Geometry: see drawing. Coordinates: mm, zero at the bounding-box minimum. A direction names the side the tool comes from. Coordinates: 2 decimals unless noted, no trailing zeros. Loops run counter-clockwise (first coordinate to the right, second up) from the corner with the lowest first, then second, coordinate; pieces in that order, holes last. Notation, with made-up numbers: (-23.5, -1.75) - (-10.5, -1.75) arc R14 ccw to (-10.5, 24.25) - close; hole circle Ø11 at (-10.75, 42). An arc over 180 degrees is marked (long way). Use a Markdown table: item, result. Add a question column.
1. Section query A-A on x = 36.65. Return the cut outline in (y, z).
2. Section query B-B on y = 26. Return the cut outline in (x, z).
3. Section query D-D on x = 21.15. Return the cut outline in (y, z), then the cut area to 3 significant figures.
4. Section query C-C on z = 36.65. Return the cut outline in (x, y).
5. Access query for the marked faces 1 and 2. Directions: +Z, -Z, +X, -X, +Y, -Y. A direction counts if a zero-diameter tool reaches every point of the face in a straight line with its end or side. Return the directions, or none.
6. Ray query, L1, parallel to Z at x = 36.65, y = 23.5; L2, parallel to X at y = 34, z = 7; L3, parallel to X at y = 23, z = 36. Return the intervals inside material, ascending. Write a range as [from, to].
7. Contact query for flat-ended pins moving along their axis: P1, Ø4, axis at x = 5.65, z = 36.65, coming from the -Y side; P2, Ø1.8, axis at x = 36.65, z = 36.65, coming from the -Y side; P3, Ø8, axis at x = 18.5, y = 11, coming from the -Z side. Output: stop coordinate, or through.
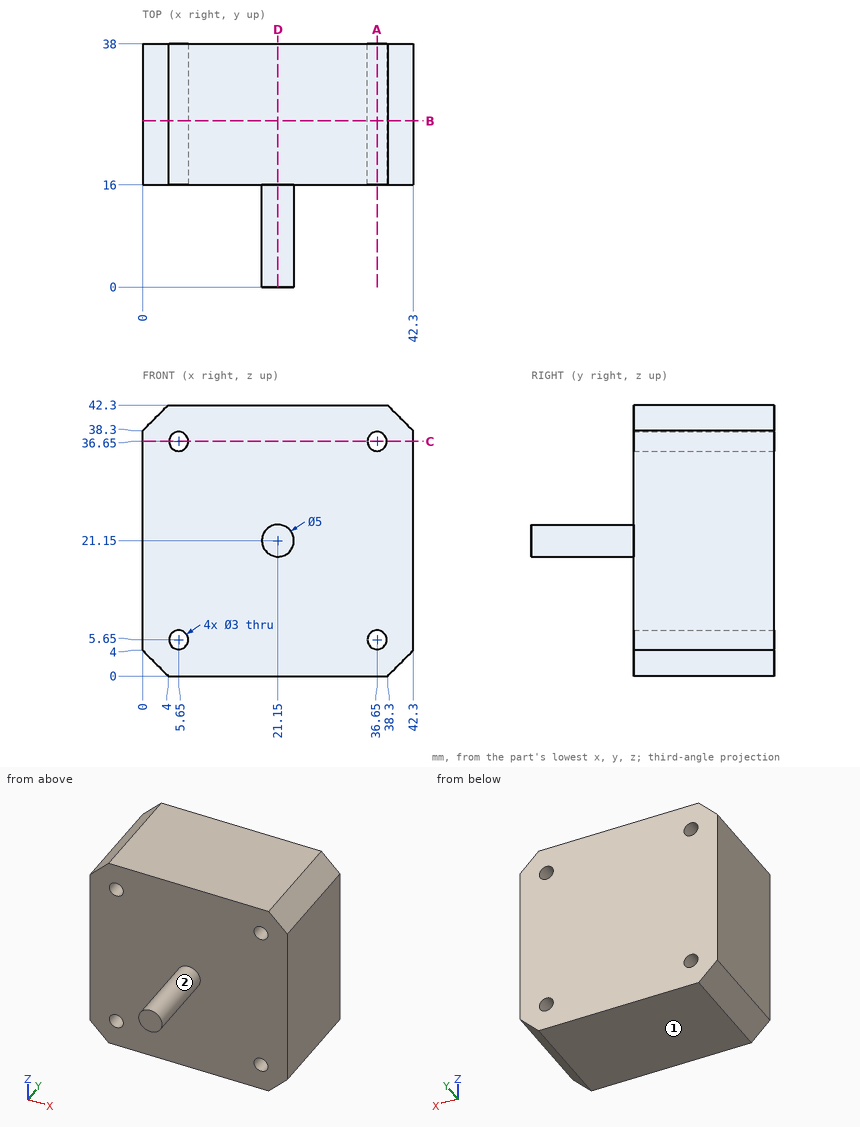
Resolved:
| question | item | result |
|---|---|---|
| 1 | outline | (16, 0) - (38, 0) - (38, 4.15) - (16, 4.15) - close; (16, 7.15) - (38, 7.15) - (38, 35.15) - (16, 35.15) - close; (16, 38.15) - (38, 38.15) - (38, 42.3) - (16, 42.3) - close |
| 2 | outline | (0, 4) - (4, 0) - (38.3, 0) - (42.3, 4) - (42.3, 38.3) - (38.3, 42.3) - (4, 42.3) - (0, 38.3) - close; hole circle Ø3 at (5.65, 5.65); hole circle Ø3 at (5.65, 36.65); hole circle Ø3 at (36.65, 5.65); hole circle Ø3 at (36.65, 36.65) |
| 3 | outline | (0, 18.65) - (16, 18.65) - (16, 0) - (38, 0) - (38, 42.3) - (16, 42.3) - (16, 23.65) - (0, 23.65) - close |
| 3 | area | 1,010 mm² |
| 4 | outline | (0, 16) - (4.15, 16) - (4.15, 38) - (0, 38) - close; (7.15, 16) - (35.15, 16) - (35.15, 38) - (7.15, 38) - close; (38.15, 16) - (42.3, 16) - (42.3, 38) - (38.15, 38) - close |
| 5 | face 1 | -Z, +X, -X, +Y, -Y |
| 5 | face 2 | -Y |
| 6 | L1 | [0, 4.15], [7.15, 35.15], [38.15, 42.3] |
| 6 | L2 | [0, 5], [6.3, 36], [37.3, 42.3] |
| 6 | L3 | [0, 4.3], [7, 35.3], [38, 42.3] |
| 7 | P1 | y = 16 |
| 7 | P2 | through |
| 7 | P3 | z = 18.65 |
